Geometry: final body of the model. Coordinates: model frame, mm. Face numbers are marked on the shaded views. A direction names the side the tool comes from. Round coordinates to 2 decimals unless told otherwise and drop trailing zeros. Loops run counter-clockwise (first coordinate to the right, second up) from the corner with the lowest first, then second, coordinate; pieces in that order, holes last. Notation, with made-up numbers: (89.5, 53.5) - (124.5, 53.5) arc R34 cw to (124.5, 84.5) - close; hole circle Ø11 at (3.5, -6). An arc over 180 degrees is marked (long way). Return JSON: item names as keys, results as strings. Group by question number.
1. Set-up query: the marked faces 3 and 4. Return all of +Z, -Z, +X, -X, +Y, -Y with unobstructed straight access to the full face (end or side cutting, diameter ignored); none if empty.
2. Section C-C on z = 8.5. Return loops of the section in (x, y).
3. Material intervals for probe 1 along Z at (x, y) = (-4.25, -10); probe 2 along Y at (x, z) = (1.5, 26); probe 3 along Z at (x, y) = (-8, -0.5), sorted ascending.
4. Section D-D on z = 40.5. Return loops of the section in (x, y), and give its area (3 significant figures).
5. Section A-A on y = 0. Return loops of the section in (x, z), and give its area (3 significant figures).
6. Draft query along X for the marked faces 1 and 2. Return one class per face: +X half, -X half, draft (parallel to the pull), parting line (faces both ways), or undercut.
7. First-contact query: pin 1 Ø8 at (x, z) = (0.5, 27.5) entering from +Y; pin 2 Ø5 at (y, z) = (-9, 29) entering from +X; pin 3 Ø1.5 at (y, z) = (-2.5, 9) entering from +X. Flat tips, straight axial feed; report the tip coordinate or a pass-through.
Autodesk Inventor part; units mm, degrees
ref_plane "YZ Plane" through (0, 0, 0) normal (1, 0, 0) x (0, 1, 0)
ref_plane "XZ Plane" through (0, 0, 0) normal (0, 1, 0) x (-1, 0, 0)
ref_plane "XY Plane" through (0, 0, 0) normal (0, 0, 1) x (1, 0, 0)
sketch "Sketch1" plane through (0, 0, 0) normal (0, 0, 1) x (1, 0, 0)
  circle A0 centre (0, 0) radius 10.16
  dimension "d0" = 20.32
extrude "Extrusion1" add sketch "Sketch1" along normal blind 4.5
sketch "Sketch2" plane through (0, 0, 4.5) normal (0, 0, 1) x (1, 0, 0)
  circle A0 centre (0, 0) radius 12
  dimension "d3" = 24
extrude "Extrusion2" add sketch "Sketch2" along normal blind 1.5
sketch "Sketch3" plane through (0, 0, 6) normal (0, 0, 1) x (1, 0, 0)
  circle A0 centre (0, 0) radius 10.5
  dimension "d6" = 21
extrude "Extrusion3" add sketch "Sketch3" along normal blind 40
sketch "Sketch5" plane through (0, 0, 46) normal (0, 0, 1) x (1, 0, 0)
  point P0 (0, 0)
sketch "Sketch6" plane through (0, 0, 46) normal (0, 0, 1) x (1, 0, 0)
  circle A0 centre (0, 0) radius 7.85
  circle A1 centre (0, 0) radius 10.5
  dimension "d25" = 15.7
  dimension "d26" = 21
extrude "Extrusion5" cut sketch "Sketch6" against normal blind 7.9
chamfer "Chamfer5" distance 1.8 angle 45 1 edges at (-10.5, 0, 38.1)
chamfer "Chamfer6" distance 5.2 distance2 3.9 1 edges at (-7.85, 0, 46) measured on face at (-0.2971, -2.4466, 46)
properties part number "objective"
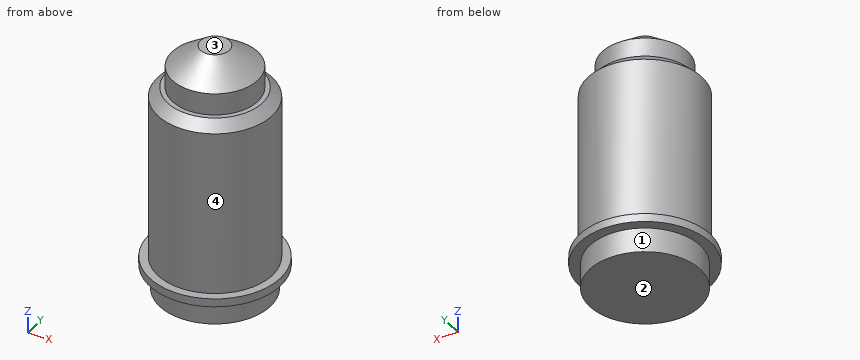
Taken from the geometry:
{
 "1": {"face 3": "+Z, +X, -X, +Y, -Y", "face 4": "+Z"},
 "2": {"outline": "circle Ø21 at (0, 0)"},
 "3": {"probe 1": "4.5 to 6", "probe 2": "-10.39 to 10.39", "probe 3": "0 to 38.1"},
 "4": {"outline": "circle Ø15.7 at (0, 0)", "area": "194 mm2"},
 "5": {"outline": "(-12, 4.5) - (-10.16, 4.5) - (-10.16, 0) - (10.16, 0) - (10.16, 4.5) - (12, 4.5) - (12, 6) - (10.5, 6) - (10.5, 36.3) - (8.7, 38.1) - (7.85, 38.1) - (7.85, 42.1) - (2.65, 46) - (-2.65, 46) - (-7.85, 42.1) - (-7.85, 38.1) - (-8.7, 38.1) - (-10.5, 36.3) - (-10.5, 6) - (-12, 6) - close", "area": "902 mm2"},
 "6": {"face 1": "parting line", "face 2": "draft"},
 "7": {"pin 1": "y = 10.5", "pin 2": "x = 8.25", "pin 3": "x = 10.35"}
}
